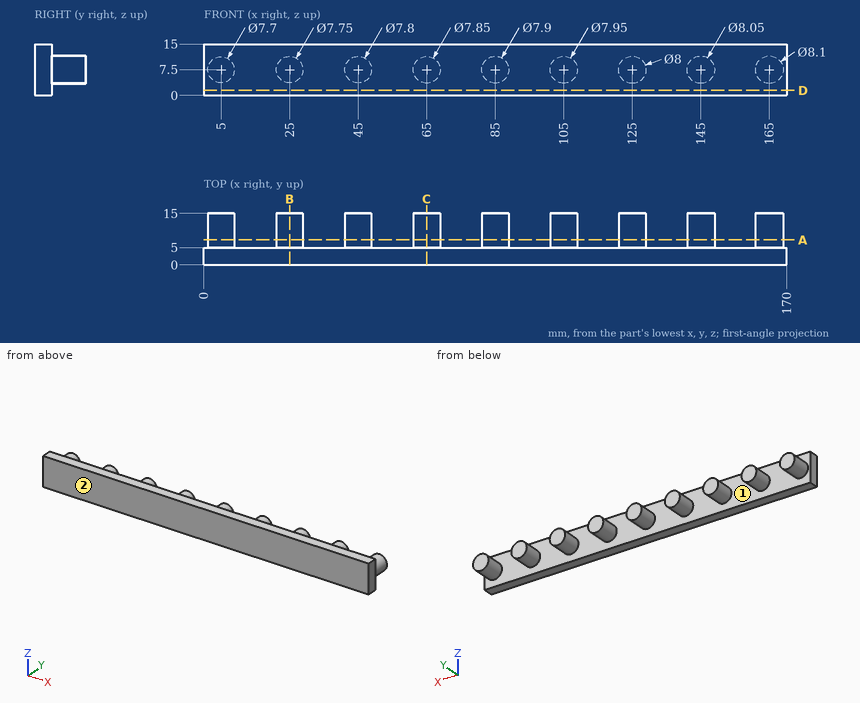
Source: three-view drawing plus pictorial views. Frame: mm from the lowest corner of the part. Coordinates: 2 decimals unless noted, no trailing zeros. Loops run counter-clockwise (first coordinate to the right, second up) from the corner with the lowest first, then second, coordinate; pieces in that order, holes last. Notation, with made-up numbers: (22, -2.75) - (77, -2.75) arc R9 ccw to (77, 7.25) - close; hole circle Ø5 at (73, -36). An arc over 180 degrees is marked (long way). Answer in a Markdown table with one row per item. Add a question column.
Item 1: Contact query for flat-ended pins moving along their axis: P1, Ø4, axis at y = 8, z = 5, coming from the +X side; P2, Ø5, axis at x = 143, y = 8.5, coming from the +Z side (3 decimals). Output: stop coordinate, or through.
Item 2: Line query: line 1 along Z through (x, y) = (44.5, 11); line 2 along Y through (x, z) = (60.5, 1.75); line 3 along Z through (x, y) = (84, 12.75). Output: solid intervals per line, ascending. Write a range as [from, to].
Item 3: Section query B-B on x = 25. Return the cut outline in (y, z) (3 decimals), then the cut area to 4 significant figures.
Item 4: Section query C-C on x = 65. Return the cut outline in (y, z) (3 decimals), then the cut area to 4 significant figures.
Item 5: Mould query, pull axis X, two halves, no side actions, for the marked faces 1 and 2. Classes: released by +X, released by -X, zero draft, split by the parting line, or undercut.
Item 6: Section query D-D on z = 1.5. Return the cut outline in (x, y), then the cut area to 3 significant figures.
Item 7: Section query A-A on y = 7.25. State how many separate pieces and enclosed holes the cut face has, then the cut area to 3 significant figures.
Recorded:
| question | item | result |
|---|---|---|
| 1 | P1 | x = 169.02 |
| 1 | P2 | z = 11.525 |
| 2 | line 1 | [3.63, 11.37] |
| 2 | line 2 | [0, 5] |
| 2 | line 3 | [3.68, 11.32] |
| 3 | outline | (0, 0) - (5, 0) - (5, 3.625) - (15, 3.625) - (15, 11.375) - (5, 11.375) - (5, 15) - (0, 15) - close |
| 3 | area | 152.5 mm^2 |
| 4 | outline | (0, 0) - (5, 0) - (5, 3.575) - (15, 3.575) - (15, 11.425) - (5, 11.425) - (5, 15) - (0, 15) - close |
| 4 | area | 153.5 mm^2 |
| 5 | face 1 | undercut |
| 5 | face 2 | zero draft |
| 6 | outline | (0, 0) - (170, 0) - (170, 5) - (0, 5) - close |
| 6 | area | 850 mm^2 |
| 7 | separate pieces | 9 |
| 7 | enclosed holes | 0 |
| 7 | area | 441 mm^2 |
